Can you work these out from the model? Positions are in its coordinate system, mm. A direction names the side the tool comes from. Round coordinates to 2 decimals unless told otherwise and drop trailing zeros. Order: outer loops, then holes, each group sorted by start corner. A loop starts at its lowest first (then second) coordinate and runs counter-clockwise, first axis right, second up. Notation, with made-up numbers: (76.5, -22) -> (126.5, -22) arc R25 cw to (126.5, 3) -> close; hole circle Ø2 at (21.5, -9). An arc over 180 degrees is marked (long way). Use a Markdown table: item, result. Add a question column.
Q1. If we section it at A-A on y = 25.5: List the corners of the cut face in (x, z) for me.
Q2. We'd pull the mould along Y, two halves only. Please class faces 4 (the face through (4.72, 22.8, 0.99)), 5 (the face through (0, 3.5, 3)), 6 (the face through (1.1, 45.04, 4.14)): +Y half, -Y half, draft (parallel to the pull), parting line (faces both ways), or undercut.
Q3. If we section it at C-C on z = 1.15: List the corners of the cut face in (x, y) for me, plus the area to 3 significant figures.
Q4. I need wall thicknesses on line 1 along X through (y, z) = (25.5, 0.5); line 2 along Z through (x, y) = (6, 6); line 3 along Y through (x, z) = (5.5, 0.3). Which ranges of each line are inside material? Lowest first, please. Write a range as [from, to].
Q5. If we section it at D-D on x = 1.5: List the corners of the cut face in (y, z) for me, plus the area to 3 significant figures.
Q6. If we section it at B-B on x = 10.5: List the corners of the cut face in (y, z) for me.
Q7. I'm going to push flat-ended pins straight in: pin 1 Ø1.5 at (x, y) = (9, 40.5) entering from +Z; pin 2 Ø1.6 at (y, z) = (18, 1) entering from -X; pin 3 Ø10.5 at (x, y) = (7.67, 25.5) entering from -Z; pin 4 Ø0.9 at (x, z) = (0.5, 3) entering from -Y. Where does each tip first touch, or does it pass through?
Q8. For faces 1 (the face through (15.8, 25, 1)), 2 (the face through (0, 47.5, 3)), 3 (the face through (0, 42.5, 3)), which set-ups out of +Z, -Z, +X, -X, +Y, -Y let a thin tool reach every point of the face, with its end or its side?
Autodesk Fusion 360 part; units mm, degrees
sketch "Sketch1" plane through (0, 0, 0) normal (0, 0, 1) x (1, 0, 0)
  line L0 (0, 0) -> (15.8, 0)
  line L1 (15.8, 0) -> (15.8, 51)
  line L2 (15.8, 51) -> (0, 51)
  line L3 (0, 51) -> (0, 0)
  dimension "d1" = 15.8
  dimension "d2" = 51
extrude "Extrude1" add sketch "Sketch1" along normal blind 2
sketch "Sketch2" plane through (0, 0, 0) normal (0, 0, -1) x (1, 0, 0)
  line L0 (0, 0) -> (0, -51)
  line L1 (0, -51) -> (15.8, -51)
  line L2 (15.8, -51) -> (15.8, 0)
  line L3 (15.8, 0) -> (0, 0)
  circle A0 centre (7.6687, -25.5) radius 4
  dimension "d5" = 8
extrude "Extrude2" cut sketch "Sketch2" against normal blind 2 contours A0
sketch "Sketch3" plane through (0, 0, 2) normal (0, 0, 1) x (-1, 0, 0)
  line L0 (0, -51) -> (0, 0)
  line L1 (0, 0) -> (-15.8, 0)
  line L2 (-15.8, 0) -> (-15.8, -51)
  line L3 (-15.8, -51) -> (0, -51)
  line L4 (0, -3.5) -> (-2, -3.5)
  line L5 (-2, -3.5) -> (-2, -8.5)
  line L6 (-2, -8.5) -> (0, -8.5)
  line L7 (0, -8.5) -> (0, -3.5)
  line L8 (0, -42.5) -> (-2, -42.5)
  line L9 (-2, -42.5) -> (-2, -47.5)
  line L10 (-2, -47.5) -> (0, -47.5)
  line L11 (0, -47.5) -> (0, -42.5)
  circle A0 centre (-7.6687, -25.5) radius 4
  dimension "d8" = 3.5
  dimension "d9" = 42.5
  dimension "d10" = 2
  dimension "d11" = 2
  dimension "d12" = 5
  dimension "d13" = 5
extrude "Extrude3" add sketch "Sketch3" along normal blind 3 contours L0 L8 L9 L10 L11 | L0 L4 L5 L6 L7
sketch "Sketch4" plane through (0, 0, 0) normal (-1, 0, 0) x (0, -1, 0)
  line L0 (-51, 0) -> (0, 0)
  line L1 (0, 0) -> (0, 2)
  line L2 (0, 2) -> (-3.5, 2)
  line L3 (-3.5, 2) -> (-3.5, 5)
  line L4 (-3.5, 5) -> (-8.5, 5)
  line L5 (-8.5, 5) -> (-8.5, 2)
  line L6 (-8.5, 2) -> (-42.5, 2)
  line L7 (-42.5, 2) -> (-42.5, 5)
  line L8 (-42.5, 5) -> (-47.5, 5)
  line L9 (-47.5, 5) -> (-47.5, 2)
  line L10 (-47.5, 2) -> (-51, 2)
  line L11 (-51, 2) -> (-51, 0)
  line L12 (-47.5, 5) -> (-42.5, 5)
  line L13 (-42.5, 5) -> (-42.5, 2)
  line L14 (-42.5, 2) -> (-47.5, 2)
  line L15 (-47.5, 2) -> (-47.5, 5)
  line L16 (-8.5, 5) -> (-3.5, 5)
  line L17 (-3.5, 5) -> (-3.5, 2)
  line L18 (-3.5, 2) -> (-8.5, 2)
  line L19 (-8.5, 2) -> (-8.5, 5)
extrude "Extrude4" add sketch "Sketch4" along normal blind 2 contours L7 L8 L9 L12 L13 L14 L15 | L3 L4 L5 L16 L17 L18 L19
fillet "Fillet1" radius 3 1 edges at (2, 6, 5)
fillet "Fillet2" radius 3 1 edges at (2, 45, 5)
chamfer "Chamfer1" distance 1.5 angle 45 1 edges at (-2, 6, 2)
chamfer "Chamfer2" distance 1.5 angle 45 1 edges at (-2, 45, 2)
Answer below:
| question | item | result |
|---|---|---|
| 1 | outline | (0, 0) -> (3.67, 0) -> (3.67, 2) -> (0, 2) -> close; (11.67, 0) -> (15.8, 0) -> (15.8, 2) -> (11.67, 2) -> close |
| 2 | face 4 | undercut |
| 2 | face 5 | -Y half |
| 2 | face 6 | draft |
| 3 | outline | (0, 0) -> (15.8, 0) -> (15.8, 51) -> (0, 51) -> close; hole circle Ø8 at (7.67, 25.5) |
| 3 | area | 756 mm² |
| 4 | line 1 | [0, 3.67], [11.67, 15.8] |
| 4 | line 2 | [0, 2] |
| 4 | line 3 | [0, 22.14], [28.86, 51] |
| 5 | outline | (0, 0) -> (51, 0) -> (51, 2) -> (47.5, 2) -> (47.5, 3.66) -> (42.5, 3.66) -> (42.5, 2) -> (8.5, 2) -> (8.5, 3.66) -> (3.5, 3.66) -> (3.5, 2) -> (0, 2) -> close |
| 5 | area | 119 mm² |
| 6 | outline | (0, 0) -> (22.67, 0) -> (22.67, 2) -> (0, 2) -> close; (28.33, 0) -> (51, 0) -> (51, 2) -> (28.33, 2) -> close |
| 7 | pin 1 | z = 2 |
| 7 | pin 2 | x = 0 |
| 7 | pin 3 | z = 0 |
| 7 | pin 4 | y = 3.5 |
| 8 | face 1 | +Z, -Z, +X, +Y, -Y |
| 8 | face 2 | +Z, +X, -X, +Y |
| 8 | face 3 | +Z, +X, -X |
